Design review of the part built by this model. Coordinates are the model's own, in mm. A direction names the side the tool comes from. Coordinates: 2 decimals unless noted, no trailing zeros. Write each loop counter-clockwise with the first axis right and the second up, starting at its lowest first coordinate (ties: lowest second). Pieces come first, ordered by that corner, then holes. Notation, with made-up numbers: M 48,18 L 66,18 A25 ccw 66,51 Z; hole C 39.5,-6.5 d4. An arc over 180 degrees is marked long. One line per question, with ' | ' between items.
from build123d import *

# Parameters (mm, degrees)
F0_W     = 38.1
F0_H     = 6.35
F1_DEPTH = 3.175
F2_R     = 1.1938
F3_DEPTH = 2.54
F4_R     = 2.54
F5_DEPTH = 18.415
F6_R     = 3.17499


# Not quite as in the source:
# - a fillet or chamfer is up to 0.001 mm smaller than in the source, because OpenCascade refuses the exact size


with BuildPart() as f1:
    # F0 (on Front) → F1 (new body)
    with BuildSketch(Plane.XZ):
        with Locations((19.05, 3.175)):
            Rectangle(F0_W, F0_H)
    extrude(amount=F1_DEPTH)

    # F2 (on face) → F3 (join)
    with BuildSketch(Plane.XZ.offset(3.175)):
        with Locations((16.51, 3.175)):
            Circle(F2_R)
        with Locations((33.02, 3.175)):
            Circle(F2_R)
    extrude(amount=F3_DEPTH)

    # F4 (on face) → F5 (join)
    with BuildSketch(Plane(origin=(0, 0, 0), x_dir=(-1, 0, 0), z_dir=(0, 1, 0))):
        with Locations((-4.8514, 3.175)):
            Circle(F4_R)
    extrude(amount=F5_DEPTH)

    # F6 (radius 3.175 in the source; OpenCascade refuses exactly that, so slightly less here)
    f6_edges = [f1.edges().sort_by_distance(p)[0] for p in [
        (38.1, -1.5875, 6.35),
        (38.1, -1.5875, 0),
        (0, -1.5875, 6.35),
        (0, -1.5875, 0),
    ]]
    fillet(f6_edges, radius=F6_R)


solid = f1.part
1. Insertion check: pin 1 Ø1.5 at (y, z) = (3, 4) entering from +X; pin 2 Ø2 at (x, z) = (19.5, 1) entering from +Y; pin 3 Ø1.5 at (y, z) = (13.5, 5) entering from +X. Each pin has a flat end and moves straight along its axis. Give the tip position at first contact, or say it passes through.
Answer sheet:
pin 1: x = 7.39 | pin 2: y = 0 | pin 3: x = 7.15
2. Take a section at C-C (y = 14.75). Write out the cut boundary in (x, z) (3 decimals), then the cut area to 3 significant figures.
Answer sheet:
outline: C 4.851,3.175 d5.08 | area: 20.3 mm^2
3. Take a section at D-D (x = 4). Write out the cut boundary in (y, z) (3 decimals).
Answer sheet:
outline: M -3.175,0 L 0,0 L 0,0.782 L 18.415,0.782 L 18.415,5.568 L 0,5.568 L 0,6.35 L -3.175,6.35 Z
4. Draft analysis for pull direction X (two halves, no side actions). For faces 4 (the face through (33, -5.715, 3)), 5 (the face through (37.15, -1.61, 5.44)), 6 (the face through (0.91, -1.61, 0.95)), 7 (the face through (17.65, -4.43, 3.53)), state which applies: pulls with the +X half, pulls with the -X half, needs draft (parallel to the pull), parting line crosses it, or undercut.
Answer sheet:
face 4: needs draft | face 5: pulls with the +X half | face 6: pulls with the -X half | face 7: undercut
5. Tool access review of faces 1 (the face through (31.827, -4.427, 3.227)), 2 (the face through (6.867, 9.079, 1.629)), 3 (the face through (16, -5.715, 3)): name each direction out of +Z, -Z, +X, -X, +Y, -Y from which nothing blocks a thin tool from reaching the whole face with its end or side.
Answer sheet:
face 1: -Y | face 2: +Y | face 3: +Z, -Z, +X, -X, -Y
6. Take a section at A-A (x = 33.02). Write out the cut boundary in (y, z) (3 decimals).
Answer sheet:
outline: M -5.715,1.981 L -3.175,1.981 L -3.175,0 L 0,0 L 0,6.35 L -3.175,6.35 L -3.175,4.369 L -5.715,4.369 Z
7. Take a section at B-B (z = 4). Write out the cut boundary in (x, y) (3 decimals).
Answer sheet:
outline: M 0.109,-3.175 L 15.647,-3.175 L 15.647,-5.715 L 17.373,-5.715 L 17.373,-3.175 L 32.157,-3.175 L 32.157,-5.715 L 33.883,-5.715 L 33.883,-3.175 L 37.991,-3.175 L 37.991,0 L 7.254,0 L 7.254,18.415 L 2.449,18.415 L 2.449,0 L 0.109,0 Z
8. To check wall thickness, follow line 1 along Y through (x, z) = (36.5, 1.25) (3 decimals); line 2 along Z through (x, y) = (5, 8.25); line 3 along X through (y, z) = (-1.5, 3.25). State the ranges of each line that lie inside material, in increasing order. Write a range as [from, to].
Answer sheet:
line 1: [-3.175, 0] | line 2: [0.64, 5.71] | line 3: [0, 38.1]
